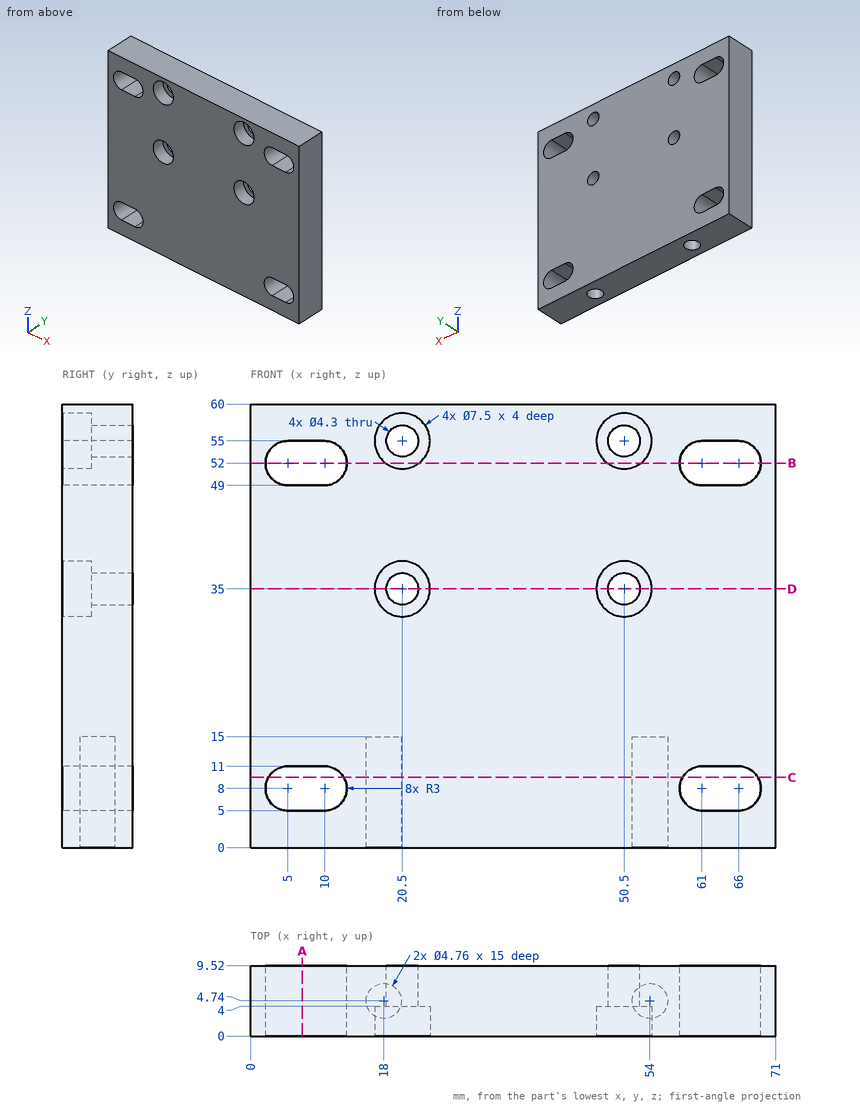
Can you work these out from the drawing? Everything is in mm from the part's minimum corner. Round coordinates to 2 decimals unless told otherwise and drop trailing zeros. Loops run counter-clockwise (first coordinate to the right, second up) from the corner with the lowest first, then second, coordinate; pieces in that order, holes last. Notation, with made-up numbers: (-11, 67) - (21, 67) arc R17 cw to (21, 85) - close; hole circle Ø10 at (79.25, -12). An arc over 180 degrees is marked (long way). Write item = value, one per line. Start each with the question number.
(1) If we section it at B-B (z = 52): Please give me the cut outline in (x, y), and give its area (3 significant figures).
(2) If we section it at D-D (z = 35): Please give me the cut outline in (x, y), and give its area (3 significant figures).
(3) If we section it at C-C (z = 9.5): Please give me the cut outline in (x, y).
(4) If we section it at A-A (x = 7): Please give me the cut outline in (y, z), and give its area (3 significant figures).
(5) For P1, Ø1.4, axis at x = 53.5, y = 4, coming from the -Z side; P2, Ø7, axis at x = 20.5, z = 35, coming from the -Y side, each with a flat end and sliding along its axis, tell me the tip position at first contact or that it passes through.
(6) If I drill on probe 1 along Z at (x, y) = (62, 1.5); probe 2 along X at (y, z) = (1.4, 35); probe 3 along Z at (x, y) = (50.5, 7.4), over which ranges is the centre line in solid material (lowest first)? Write a range as [from, to].
Ans:
q1.outline = (0, 0) - (2, 0) - (2, 9.52) - (0, 9.52) - close; (13, 0) - (18.25, 0) - (18.25, 4) - (22.75, 4) - (22.75, 0) - (48.25, 0) - (48.25, 4) - (52.75, 4) - (52.75, 0) - (58, 0) - (58, 9.52) - (13, 9.52) - close; (69, 0) - (71, 0) - (71, 9.52) - (69, 9.52) - close
q1.area = 430 mm²
q2.outline = (0, 0) - (16.75, 0) - (16.75, 4) - (18.35, 4) - (18.35, 9.52) - (0, 9.52) - close; (22.65, 4) - (24.25, 4) - (24.25, 0) - (46.75, 0) - (46.75, 4) - (48.35, 4) - (48.35, 9.52) - (22.65, 9.52) - close; (52.65, 4) - (54.25, 4) - (54.25, 0) - (71, 0) - (71, 9.52) - (52.65, 9.52) - close
q2.area = 568 mm²
q3.outline = (0, 0) - (2.4, 0) - (2.4, 9.52) - (0, 9.52) - close; (12.6, 0) - (58.4, 0) - (58.4, 9.52) - (12.6, 9.52) - close; (68.6, 0) - (71, 0) - (71, 9.52) - (68.6, 9.52) - close; hole circle Ø4.76 at (18, 4.74); hole circle Ø4.76 at (54, 4.74)
q4.outline = (0, 0) - (9.52, 0) - (9.52, 5) - (0, 5) - close; (0, 11) - (9.52, 11) - (9.52, 49) - (0, 49) - close; (0, 55) - (9.52, 55) - (9.52, 60) - (0, 60) - close
q4.area = 457 mm²
q5.P1 = 15
q5.P2 = 4
q6.probe_1 = [0, 5], [11, 49], [55, 60]
q6.probe_2 = [0, 16.75], [24.25, 46.75], [54.25, 71]
q6.probe_3 = [0, 32.85], [37.15, 52.85], [57.15, 60]
